Read the model definition and answer for the solid it produces. Units are mm, in the model's axes. A direction names the side the tool comes from. Give positions to 0.01 mm unless a question says otherwise; leave off trailing zeros. Order: outer loops, then holes, each group sorted by start corner. A loop starts at its lowest first (then second) coordinate and runs counter-clockwise, first axis right, second up. Notation, with made-up numbers: (21, 10) - (46, 10) arc R13 cw to (46, 18) - close; hole circle Ø10 at (58, 88.5). An arc over 180 degrees is marked (long way). Use a Markdown table: item, result. Add a question column.
1. A flat-ended cylindrical pin translates along its axis: P1, Ø1.5, axis at y = 1, z = 5.5, coming from the -X side. Find the tip coordinate at first contact, or state that the pin passes through.
2. Consider L1, parallel to Z at x = 0.55, y = 0.8; L2, parallel to X at y = 1.3, z = 1.75; L3, parallel to Z at x = -0.1, y = -1.25. Determine where each line is inside the solid, lowest interval first.
3. A cutting plane is placed at D-D on z = 11. Determine the outline of the cut face in (x, y).
4. A cutting plane is placed at C-C on z = -3. Determine the outline of the cut face in (x, y), and give its area (3 significant figures).
5. Which of the six approach directions +Z, -Z, +X, -X, +Y, -Y give full straight-line access (tool end or side, diameter ignored) to faces 1 (the cylindrical face through (-0.75, 0.03, 10.97)), 2 (the flat face through (0, 0, 13)), 3 (the cylindrical face through (0, -1, -2))?
6. A cutting plane is placed at A-A on x = 0. Determine the outline of the cut face in (y, z).
```python
from build123d import *

# Parameters (mm, degrees)
F0_R     = 1.5
F1_DEPTH = 9
F2_R     = 0.75
F3_DEPTH = 4
F4_R     = 1
F5_DEPTH = 5


with BuildPart() as f1:
    # F0 (on Top) → F1 (new body)
    with BuildSketch(Plane.XY):
        Circle(F0_R)
    extrude(amount=F1_DEPTH)

    # F2 (on face) → F3 (join)
    with BuildSketch(Plane.XY.offset(9)):
        Circle(F2_R)
    extrude(amount=F3_DEPTH)

    # F4 (on Top) → F5 (join)
    with BuildSketch(Plane.XY):
        Circle(F4_R)
    extrude(amount=-F5_DEPTH)


solid = f1.part
```
Output values:
| question | item | result |
|---|---|---|
| 1 | P1 | x = -1.48 |
| 2 | L1 | -5 to 9 |
| 2 | L2 | -0.75 to 0.75 |
| 2 | L3 | 0 to 9 |
| 3 | outline | circle Ø1.5 at (0, 0) |
| 4 | outline | circle Ø2 at (0, 0) |
| 4 | area | 3.14 mm² |
| 5 | face 1 | +Z |
| 5 | face 2 | +Z, +X, -X, +Y, -Y |
| 5 | face 3 | -Z |
| 6 | outline | (-1.5, 0) - (-1, 0) - (-1, -5) - (1, -5) - (1, 0) - (1.5, 0) - (1.5, 9) - (0.75, 9) - (0.75, 13) - (-0.75, 13) - (-0.75, 9) - (-1.5, 9) - close |
